```python
from build123d import *

# Parameters (mm, degrees)
SKETCH1_R            = 7.62
SKETCH1_R_2          = 6.096
BOSS_EXTRUDE1_DEPTH  = 10.16
SKETCH1_4_R          = 12.065
SKETCH1_4_R_2        = 7.62
BOSS_EXTRUDE2_DEPTH  = 12.7
SKETCH9_R            = 12.065
SKETCH9_R_2          = 7.62
BOSS_EXTRUDE22_DEPTH = 1.27
SKETCH10_R           = 8.89
SKETCH10_R_2         = 7.62
CUT_EXTRUDE5_DEPTH   = 3.81
SKETCH14_W           = 4.826
SKETCH14_H           = 8.001
CUT_EXTRUDE8_DEPTH   = 7.62
CUT_EXTRUDE9_DEPTH   = 5.08
SKETCH16_R           = 12.065
BOSS_EXTRUDE24_DEPTH = 3.175
SKETCH17_R           = 7.366
SKETCH17_R_2         = 6.096
CUT_EXTRUDE10_DEPTH  = 5.08
CUT_EXTRUDE11_DEPTH  = 8.255


with BuildPart() as part:
    # Sketch1 → Boss-Extrude1 (new body)
    with BuildSketch(Plane(origin=(0, 0, 0), x_dir=(1, 0, 0), z_dir=(0, 1, 0))):
        Circle(SKETCH1_R)
        Circle(SKETCH1_R_2, mode=Mode.SUBTRACT)
    extrude(amount=BOSS_EXTRUDE1_DEPTH)

    # Sketch1<4> → Boss-Extrude2 (add)
    with BuildSketch(Plane(origin=(0, 0, 0), x_dir=(1, 0, 0), z_dir=(0, 1, 0))):
        Circle(SKETCH1_4_R)
        Circle(SKETCH1_4_R_2, mode=Mode.SUBTRACT)
    extrude(amount=BOSS_EXTRUDE2_DEPTH)

    # Sketch9 → Boss-Extrude22 (add)
    with BuildSketch(Plane(origin=(0, 12.7, 0), x_dir=(1, 0, 0), z_dir=(0, 1, 0))):
        Circle(SKETCH9_R)
        Circle(SKETCH9_R_2, mode=Mode.SUBTRACT)
    extrude(amount=BOSS_EXTRUDE22_DEPTH)

    # Sketch10 → Cut-Extrude5 (cut)
    with BuildSketch(Plane(origin=(0, 13.97, 0), x_dir=(1, 0, 0), z_dir=(0, 1, 0))):
        Circle(SKETCH10_R)
        Circle(SKETCH10_R_2, mode=Mode.SUBTRACT)
    extrude(amount=-CUT_EXTRUDE5_DEPTH, mode=Mode.SUBTRACT)

    # Sketch14 → Cut-Extrude8 (cut)
    with BuildSketch(Plane.XZ):
        with Locations((0, -4.0005)):
            Rectangle(SKETCH14_W, SKETCH14_H)
    extrude(amount=-CUT_EXTRUDE8_DEPTH, mode=Mode.SUBTRACT)

    # Sketch15 → Cut-Extrude9 (cut)
    with BuildSketch(Plane.XZ.offset(-7.62)):
        with BuildLine():
            Line((2.413, -8.001), (-2.413, -8.001))
            ThreePointArc((-2.413, -8.001), (0, -10.033), (2.413, -8.001))
        make_face()
    extrude(amount=CUT_EXTRUDE9_DEPTH, mode=Mode.SUBTRACT)

    # Sketch16 → Boss-Extrude24 (add)
    with BuildSketch(Plane.XZ):
        Circle(SKETCH16_R)
        with BuildLine():
            Line((2.413, -5.598093), (2.413, -8.001))
            Line((2.413, -8.001), (-2.413, -8.001))
            Line((-2.413, -8.001), (-2.413, -5.598093))
            ThreePointArc((-2.413, -5.598093), (0, 6.096), (2.413, -5.598093))
        make_face(mode=Mode.SUBTRACT)
    extrude(amount=BOSS_EXTRUDE24_DEPTH)

    # Sketch17 → Cut-Extrude10 (cut)
    with BuildSketch(Plane(origin=(0, 10.16, 0), x_dir=(1, 0, 0), z_dir=(0, 1, 0))):
        Circle(SKETCH17_R)
        Circle(SKETCH17_R_2, mode=Mode.SUBTRACT)
    extrude(amount=-CUT_EXTRUDE10_DEPTH, mode=Mode.SUBTRACT)

    # Sketch18 → Cut-Extrude11 (cut)
    with BuildSketch(Plane(origin=(0, 5.08, 0), x_dir=(1, 0, 0), z_dir=(0, 1, 0))):
        with BuildLine():
            Line((0, 0), (-7.11501, -1.906461))
            ThreePointArc((-7.11501, -1.906461), (-7.366, 0), (-7.11501, 1.906461))
            Line((-7.11501, 1.906461), (0, 0))
        make_face()
    extrude(amount=-CUT_EXTRUDE11_DEPTH, mode=Mode.SUBTRACT)


solid = part.part
```
Design review of the part built by this model. Coordinates are the model's own, in mm. A direction names the side the tool comes from. Round coordinates to 2 decimals unless told otherwise and drop trailing zeros. Write each loop counter-clockwise with the first axis right and the second up, starting at its lowest first coordinate (ties: lowest second). Pieces come first, ordered by that corner, then holes. Notation, with made-up numbers: (-20, 25.5) -> (31, 25.5) arc R25 cw to (31, 54.5) -> close; hole circle Ø10 at (80, 19.5). An arc over 180 degrees is marked (long way). Write item = value, one per line. Start each with the question number.
1) Take a section at B-B, the plane z = 0. State the section outline as (x, y) points (3 decimals).
2) Take a section at A-A, the plane x = 0. State the section outline as (y, z) points (3 decimals), plus the area to 3 significant figures.
3) Clearance check with flat-ended pins moving along their axes: pin 1 (3 mm diameter, centred on y = -1.5, z = 8.5, fed in from -X); pin 2 (8 mm diameter, centred on x = 9.5, y = 10.5, fed in from -Z); pin 3 (3 mm diameter, centred on x = 7.5, y = 2.5, fed in from -Z). State where each tip first meets the part, or that it passes through.
4) Tool access review of faces 4 (the face through (0, 0, -8.001)), 5 (the face through (-5, 5.08, -4)), 6 (the face through (-6.51, 1.01, -1.744)), 7 (the face through (0, 2.54, -9)): name each direction out of +Z, -Z, +X, -X, +Y, -Y from which nothing blocks a thin tool from reaching the whole face with its end or side.
5) Take a section at C-C, the plane y = 6.25. State the section outline as (x, z) points (3 decimals), plus the area to 3 significant figures.
6) Take a section at D-D, the plane x = 6.5. State the section outline as (y, z) points (3 decimals).
7) Wall thickness on probe 1 along Z at (x, y) = (0, -1.25) (3 decimals); probe 2 along X at (y, z) = (-0.55, 0) (3 decimals); probe 3 along Y at (x, z) = (7.25, 4) (3 decimals): over which ranges is each line inside the solid? List them lowest first. Write a range as from..to.
8) Mouldability with a two-part tool opening along Y and no side actions: class faces 1 (the face through (11.51, 5.52, 3.62)), 2 (the face through (-3, -3.175, 6)), 3 (the face through (0, 7.62, -8)) as +Y half, -Y half, draft (parallel to the pull), parting line (faces both ways), or undercut.
Results list:
q1.outline = (-12.065, -3.175) -> (-7.366, -3.175) -> (-7.366, 10.16) -> (-8.89, 10.16) -> (-8.89, 13.97) -> (-12.065, 13.97) -> close; (6.096, -3.175) -> (12.065, -3.175) -> (12.065, 13.97) -> (8.89, 13.97) -> (8.89, 10.16) -> (7.366, 10.16) -> (7.366, 5.08) -> (6.096, 5.08) -> close
q2.outline = (-3.175, -12.065) -> (13.97, -12.065) -> (13.97, -8.89) -> (10.16, -8.89) -> (10.16, -7.366) -> (7.62, -7.366) -> (7.62, -10.033) -> (2.54, -10.033) -> (2.54, -8.001) -> (-3.175, -8.001) -> close; (-3.175, 6.096) -> (5.08, 6.096) -> (5.08, 7.366) -> (10.16, 7.366) -> (10.16, 8.89) -> (13.97, 8.89) -> (13.97, 12.065) -> (-3.175, 12.065) -> close
q2.area = 143 mm²
q3.pin_1 = -9.83
q3.pin_2 = -10.74
q3.pin_3 = -10.47
q4.face_4 = -Y
q4.face_5 = +Y
q4.face_6 = +Y, -Y
q4.face_7 = none
q5.outline = circle Ø24.13 at (0, 0); hole (-2.413, -8.001) arc R2.449 ccw to (2.413, -8.001) -> (2.413, -6.96) arc R7.366 ccw (long way) to (-2.413, -6.96) -> close
q5.area = 276 mm²
q6.outline = (-3.175, -10.164) -> (13.97, -10.164) -> (13.97, -6.065) -> (10.16, -6.065) -> (10.16, -3.465) -> (5.08, -3.465) -> (5.08, 3.465) -> (10.16, 3.465) -> (10.16, 6.065) -> (13.97, 6.065) -> (13.97, 10.164) -> (-3.175, 10.164) -> close
q7.probe_1 = -12.065..-8.001, 6.096..12.065
q7.probe_2 = -12.065..-7.366, 6.096..12.065
q7.probe_3 = -3.175..10.16
q8.face_1 = draft
q8.face_2 = -Y half
q8.face_3 = undercut
